The listing builds one solid part. Answer for the finished solid, in the listing's coordinates (mm). Give positions to 0.01 mm unless a question says otherwise; leave off trailing zeros. Loops run counter-clockwise (first coordinate to the right, second up) from the corner with the lowest first, then second, coordinate; pieces in that order, holes last. Notation, with made-up numbers: M 9,63 L 26,63 A20 cw 26,78 Z; hole C 44.5,45.25 d10. An arc over 180 degrees is marked long. Return JSON: item names as keys, results as strings.
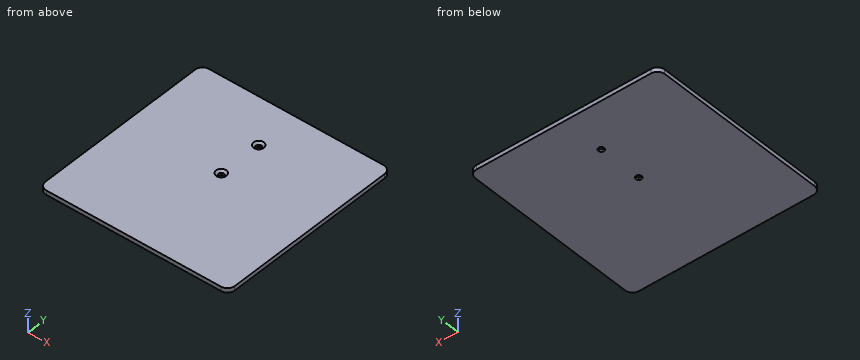
from build123d import *

# Parameters (mm, degrees)
F0_W           = 130
F0_H           = 130
F1_DEPTH       = 3
F2_D           = 4
F2_CSINK_D     = 7
F2_CSINK_ANGLE = 90
F3_R           = 5


with BuildPart() as f1:
    # F0 (on Top) → F1 (new body)
    with BuildSketch(Plane.XY):
        Rectangle(F0_W, F0_H)
    extrude(amount=-F1_DEPTH)

    # F2 (through all)
    with Locations(Plane.XY):
        with Locations((0, 35), (0, 5)):
            CounterSinkHole(F2_D / 2, F2_CSINK_D / 2, counter_sink_angle=F2_CSINK_ANGLE)

    # F3
    f3_edges = [f1.edges().sort_by_distance(p)[0] for p in [
        (-65, 65, -1.5),
        (65, 65, -1.5),
        (65, -65, -1.5),
        (-65, -65, -1.5),
    ]]
    fillet(f3_edges, radius=F3_R)


solid = f1.part
(1) Straight lines are drawn through the part: line 1 along Y through (x, z) = (0, -2.4); line 2 along X through (y, z) = (35, -2.55). For each, find the intervals that lie inside material, in ascending order.
Values follow:
{"line 1": "-65 to 3, 7 to 33, 37 to 65", "line 2": "-65 to -2, 2 to 65"}
(2) The part is cut by section A-A (y = 35). Determine the outline of the cut face in (x, z), and give its area (3 significant figures).
Values follow:
{"outline": "M -65,-3 L -2,-3 L -2,-1.5 L -3.5,0 L -65,0 Z; M 2,-3 L 65,-3 L 65,0 L 3.5,0 L 2,-1.5 Z", "area": "376 mm²"}
(3) The part is cut by section B-B (x = 0). Determine the outline of the cut face in (y, z).
Values follow:
{"outline": "M -65,-3 L 3,-3 L 3,-1.5 L 1.5,0 L -65,0 Z; M 7,-3 L 33,-3 L 33,-1.5 L 31.5,0 L 8.5,0 L 7,-1.5 Z; M 37,-3 L 65,-3 L 65,0 L 38.5,0 L 37,-1.5 Z"}
(4) Given pin 1 (6.5 mm diameter, centred on x = 0, y = 5, fed in from +Z), flat-ended and moving along its own axis, determine where the tip first touches the part or whether it passes through.
Values follow:
{"pin 1": "z = -0.25"}
